from build123d import *

# Parameters (mm, degrees)
F0_R     = 1
F0_R_2   = 1.524
F1_DEPTH = 2.54


with BuildPart() as f1:
    # F0 (on Top) → F1 (new body)
    with BuildSketch(Plane.XY):
        with BuildLine():
            Line((6.35, -19.05), (6.35, 19.05))
            ThreePointArc((6.35, 19.05), (4.490128, 23.540128), (0, 25.4))
            ThreePointArc((0, 25.4), (-4.490128, 23.540128), (-6.35, 19.05))
            Line((-6.35, 19.05), (-6.35, -19.05))
            ThreePointArc((-6.35, -19.05), (-4.490128, -23.540128), (0, -25.4))
            ThreePointArc((0, -25.4), (4.490128, -23.540128), (6.35, -19.05))
        make_face()
        with Locations((0, -23.6601)):
            Circle(F0_R, mode=Mode.SUBTRACT)
        with Locations((0, -19.05)):
            Circle(F0_R_2, mode=Mode.SUBTRACT)
        with Locations((0, -14.4399)):
            Circle(F0_R, mode=Mode.SUBTRACT)
        with Locations((0, 19.05)):
            Circle(F0_R_2, mode=Mode.SUBTRACT)
    extrude(amount=F1_DEPTH)


solid = f1.part
Read the model definition and answer for the solid it produces. Units are mm, in the model's axes. Give positions to 0.01 mm unless a question says otherwise; leave off trailing zeros. Loops run counter-clockwise (first coordinate to the right, second up) from the corner with the lowest first, then second, coordinate; pieces in that order, holes last. Notation, with made-up numbers: M 35,54 L 75,54 A25 ccw 75,86 Z; hole C 29,42 d10. An arc over 180 degrees is marked long. Write each question's results on one line, items separated by ' | '.
1. Section C-C on x = 5 is taken. Give the vertices of the cut face in (y, z), plus the area to 3 significant figures.
Values:
outline: M -22.96,0 L 22.96,0 L 22.96,2.54 L -22.96,2.54 Z | area: 117 mm^2
2. Section B-B on z = 1.1 is taken. Give the vertices of the cut face in (x, y), plus the area to 3 significant figures.
Values:
outline: M -6.35,-19.05 A6.35 ccw 6.35,-19.05 L 6.35,19.05 A6.35 ccw -6.35,19.05 Z; hole C 0,-19.05 d3.05; hole C 0,19.05 d3.05; hole C 0,-23.66 d2; hole C 0,-14.44 d2 | area: 590 mm^2
3. The mould has two halves that part along X. Classify faces 1 (the face through (-0.33, -20.538, 1.252)), 2 (the face through (6.35, 0, 1)), 3 (the face through (0, 0, 0)): pulls with the +X half, pulls with the -X half, needs draft (parallel to the pull), parting line crosses it, or undercut.
Values:
face 1: undercut | face 2: pulls with the +X half | face 3: needs draft
4. Straight lines are drawn through the part: line 1 (Y direction, x = 0.75, z = 2.05); line 2 (Y direction, x = -2, z = 0.85); line 3 (Y direction, x = -4, z = 0.65). For each, find the intervals that lie inside material, in ascending order. Write a range as [from, to].
Values:
line 1: y = [-25.36, -24.32], [-23, -20.38], [-17.72, -15.1], [-13.78, 17.72], [20.38, 25.36] | line 2: y = [-25.08, 25.08] | line 3: y = [-23.98, 23.98]
5. Section A-A on x = -0.5 is taken. Give the vertices of the cut face in (y, z), plus the area to 3 significant figures.
Values:
outline: M -25.38,0 L -24.53,0 L -24.53,2.54 L -25.38,2.54 Z; M -22.79,0 L -20.49,0 L -20.49,2.54 L -22.79,2.54 Z; M -17.61,0 L -15.31,0 L -15.31,2.54 L -17.61,2.54 Z; M -13.57,0 L 17.61,0 L 17.61,2.54 L -13.57,2.54 Z; M 20.49,0 L 25.38,0 L 25.38,2.54 L 20.49,2.54 Z | area: 106 mm^2
